```python
from build123d import *

# Parameters (mm, degrees)
SKETCH1_R           = 7.5
BOSS_EXTRUDE1_DEPTH = 50
SKETCH2_W           = 5
SKETCH2_H           = 5
CUT_EXTRUDE1_DEPTH  = 10
FILLET1_R           = 2.5
FILLET2_R           = 2.5
CUT_EXTRUDE2_START  = -15
CUT_EXTRUDE2_DEPTH  = 15


with BuildPart() as part:
    # Sketch1 → Boss-Extrude1 (new, symmetric)
    with BuildSketch(Plane.XY):
        Circle(SKETCH1_R)
    extrude(amount=BOSS_EXTRUDE1_DEPTH, both=True)

    # Sketch2 → Cut-Extrude1 (cut, symmetric)
    with BuildSketch(Plane.XY):
        with Locations((0, 7)):
            Rectangle(SKETCH2_W, SKETCH2_H)
    extrude(amount=CUT_EXTRUDE1_DEPTH, both=True, mode=Mode.SUBTRACT)

    # Fillet1
    fillet1_edges = [part.edges().sort_by_distance(p)[0] for p in [
        (-2.5, 5.785533906, -10),
        (2.5, 5.785533906, -10),
    ]]
    fillet(fillet1_edges, radius=FILLET1_R - 0.0001)  # a hair under: the kernel refuses the full size

    # Fillet2
    fillet2_edges = [part.edges().sort_by_distance(p)[0] for p in [
        (-2.5, 5.785533906, 10),
        (2.5, 5.785533906, 10),
    ]]
    fillet(fillet2_edges, radius=FILLET2_R - 0.0001)  # a hair under: the kernel refuses the full size

    # Sketch3 → Cut-Extrude2 (cut)
    with BuildSketch(Plane(origin=(0, 0, -50), x_dir=(-1, 0, 0), z_dir=(0, 0, -1)).offset(CUT_EXTRUDE2_START)):
        with BuildLine():
            Line((-3.741657387, 6.5), (3.741657387, 6.5))
            ThreePointArc((3.741657387, 6.5), (0, 7.5), (-3.741657387, 6.5))
        make_face()
        with BuildLine():
            Line((6.5, -3.741657387), (6.5, 3.741657387))
            ThreePointArc((6.5, 3.741657387), (7.5, 0), (6.5, -3.741657387))
        make_face()
    extrude(amount=CUT_EXTRUDE2_DEPTH, mode=Mode.SUBTRACT)


solid = part.part
```
Can you work these out from the model? Positions are in its coordinate system, mm. A direction names the side the tool comes from. Round coordinates to 2 decimals unless told otherwise and drop trailing zeros. Loops run counter-clockwise (first coordinate to the right, second up) from the corner with the lowest first, then second, coordinate; pieces in that order, holes last. Notation, with made-up numbers: M 21,79 L 52,79 A13 cw 52,84 Z; hole C 66.25,71.5 d3. An arc over 180 degrees is marked long. Write item = value, one per line. Start each with the question number.
(1) Which directions (+Z, -Z, +X, -X, +Y, -Y) give clear straight access to the entire face, cutting with the end or side of a thin tool? Please do faces 1 (the face through (2, 6, 9)), 2 (the face through (0, 0, 50)), 3 (the face through (-6.5, 0, -42)).
(2) Suppose I cut it at A-A on z = 0.5. Write out the boundary of the cut face in (x, y), plus the area to 3 significant figures.
(3) Suppose I cut it at B-B on x = -5.5. Write out the boundary of the cut face in (y, z).
(4) If we mould it in two halves opening along X, with no side actions, what happens to faces 4 (the face through (3.461, -6.654, 0.7)), 5 (the face through (-2, 6, -9)), 6 (the face through (0, 6.5, -42))? For each: released by +X, released by -X, zero draft, split by the parting line, or undercut.
(5) Suppose I cut it at C-C on z = -19. Write out the boundary of the cut face in (x, y), plus the area to 3 significant figures.
(6) I need wall thicknesses on line 1 along Z through (x, y) = (0.25, 6.25); line 2 along Y through (x, z) = (-2.25, -31); line 3 along Y through (x, z) = (-4, 32.5). Which ranges of each line are inside material? Lowest first, please.
(7) I'm going to push flat-ended pins straight in: P1, Ø1.5, axis at y = 1.5, z = 35, coming from the +X side; P2, Ø0.8, axis at x = -7, y = -0.5, coming from the -Z side; P3, Ø8, axis at x = 2, z = -45, coming from the +Y side. Where does each tip first touch, or does it pass through?
Answer block:
q1.face_1 = +Y
q1.face_2 = +Z, +X, -X, +Y, -Y
q1.face_3 = -Z, -X, +Y, -Y
q2.outline = M -2.5,4.5 L -2.5,7.07 A7.5 ccw long 2.5,7.07 L 2.5,4.5 Z
q2.area = 162 mm²
q3.outline = M -5.1,-50 L 5.1,-50 L 5.1,50 L -5.1,50 Z
q4.face_4 = split by the parting line
q4.face_5 = undercut
q4.face_6 = zero draft
q5.outline = C 0,0 d15
q5.area = 177 mm²
q6.line_1 = -50 to -9.99, 9.99 to 50
q6.line_2 = -7.15 to 7.15
q6.line_3 = -6.34 to 6.34
q7.P1 = 7.46
q7.P2 = -35
q7.P3 = 6.5
